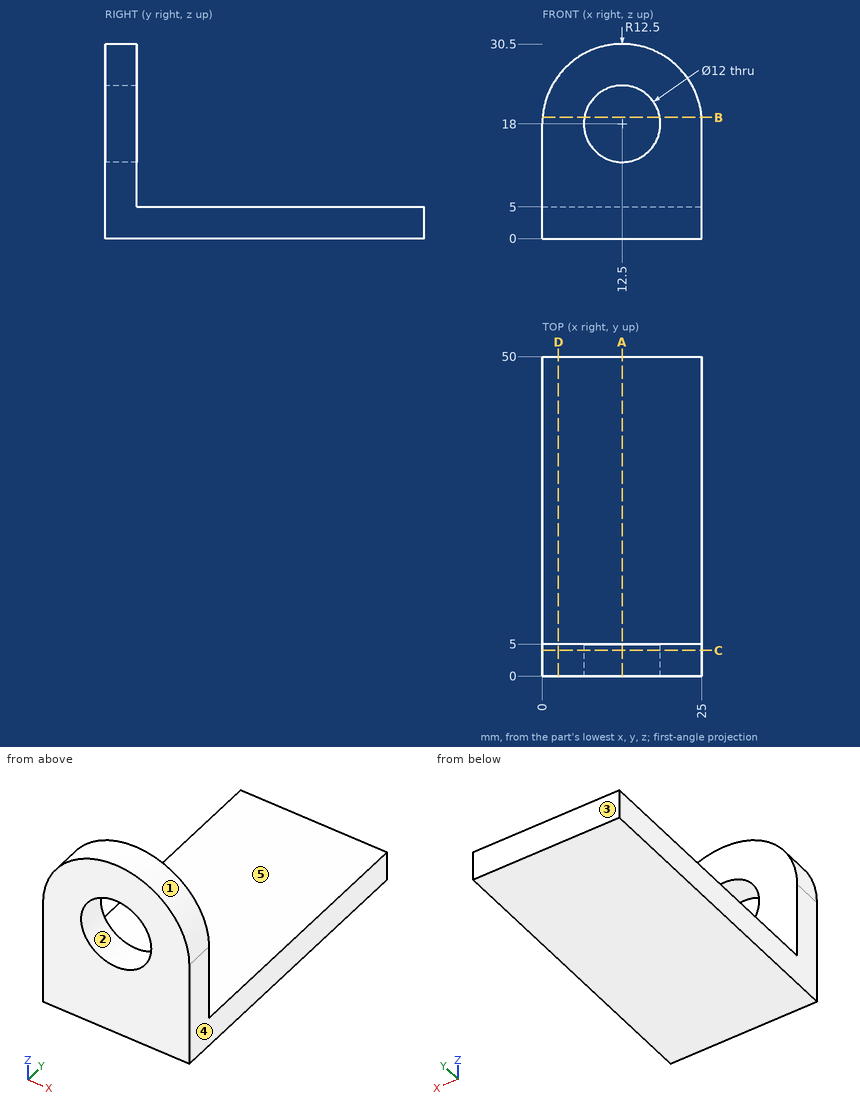
The drawing under review shows one solid part. Ordinate dimensions are in mm from its lowest x, y, z. A direction names the side the tool comes from. Give positions to 0.01 mm unless a question says otherwise; leave off trailing zeros. Write each loop counter-clockwise with the first axis right and the second up, starting at its lowest first coordinate (ties: lowest second). Pieces come first, ordered by that corner, then holes. Notation, with made-up numbers: M -24,12.25 L -20,12.25 A31 ccw -20,46.25 Z; hole C 51.25,36 d4. An arc over 180 degrees is marked long. Write each question's results on one line, items separated by ' | '. Start each with the question number.
1. For the marked faces 4 and 5, list the 3-axis set-ups (+Z, -Z, +X, -X, +Y, -Y) from which the entire face can be reached by the end or side of a thin tool; tool diameter is ignored.
2. We need section A-A (x = 12.5). Write out the cut boundary in (y, z).
3. We need section C-C (y = 4). Write out the cut boundary in (x, z).
4. We need section D-D (x = 2.5). Write out the cut boundary in (y, z).
5. We need section B-B (z = 19). Write out the cut boundary in (x, y).
6. Mouldability with a two-part tool opening along X and no side actions: class the marked faces 1, 2 and 3 as released by +X, released by -X, zero draft, split by the parting line, or undercut.
7. For probe 1 along Z at (x, y) = (12.5, 3.35); probe 2 along Y at (x, z) = (6.5, 28.5), list the stretches that pass through material, from the lowest coordinate up. Write a range as [from, to].
8. Insertion check: pin 1 Ø1 at (x, z) = (18, 24.5) entering from +Y; pin 2 Ø2 at (x, y) = (7, 19) entering from +Z. Each pin has a flat end and moves straight along its axis. Give the tip position at first contact, or say it passes through.
Results found:
1) face 4: +Z, -Z, +X, +Y, -Y | face 5: +Z, +X, -X, +Y
2) outline: M 0,0 L 50,0 L 50,5 L 5,5 L 5,12 L 0,12 Z; M 0,24 L 5,24 L 5,30.5 L 0,30.5 Z
3) outline: M 0,0 L 25,0 L 25,18 A12.5 ccw 0,18 Z; hole C 12.5,18 d12
4) outline: M 0,0 L 50,0 L 50,5 L 5,5 L 5,25.5 L 0,25.5 Z
5) outline: M 0.04,0 L 6.58,0 L 6.58,5 L 0.04,5 Z; M 18.42,0 L 24.96,0 L 24.96,5 L 18.42,5 Z
6) face 1: split by the parting line | face 2: undercut | face 3: zero draft
7) probe 1: z = [0, 12], [24, 30.5] | probe 2: y = [0, 5]
8) pin 1: stops at y = 5 | pin 2: stops at z = 5
